Autodesk Inventor part; units mm, degrees
ref_plane "YZ Plane" through (0, 0, 0) normal (1, 0, 0) x (0, 1, 0)
ref_plane "XZ Plane" through (0, 0, 0) normal (0, 1, 0) x (-1, 0, 0)
ref_plane "XY Plane" through (0, 0, 0) normal (0, 0, 1) x (1, 0, 0)
sketch "main" plane through (0, 0, 0) normal (0, 0, 1) x (1, 0, 0)
  line L0 (-49.2738, 43.4655) -> (65.0262, 43.4655)
  circle A0 centre (65.0262, 37.1155) radius 2.1844
  line L1 (71.3762, 37.1155) -> (71.3762, 32.7721)
  arc A1 (71.3762, 37.1155) -> (65.0262, 43.4655) centre (65.0262, 37.1155) ccw
  line L2 (-71.4988, 29.5971) -> (-102.2861, 29.5971)
  line L3 (-105.3112, 25.4581) -> (-94.5785, -8.22)
  line L4 (-58.7988, 29.5971) -> (118.0384, 29.5971)
  line L5 (121.0635, 25.4581) -> (110.3309, -8.22)
  line L6 (101.2556, -14.8529) -> (-85.5032, -14.8529)
  arc A2 (-94.5785, -8.22) -> (-85.5032, -14.8529) centre (-85.5032, -5.3279) ccw
  arc A3 (101.2556, -14.8529) -> (110.3309, -8.22) centre (101.2556, -5.3279) ccw
  arc A4 (-102.2861, 29.5971) -> (-105.3112, 25.4581) centre (-102.2861, 26.4221) ccw
  arc A5 (121.0635, 25.4581) -> (118.0384, 29.5971) centre (118.0384, 26.4221) ccw
  arc A6 (71.3762, 32.7721) -> (74.5512, 29.5971) centre (74.5512, 32.7721) ccw
  line L7 (-58.7988, 29.5971) -> (-71.4988, 29.5971)
  circle A7 centre (-49.2738, 37.1155) radius 2.1844
  arc A8 (-49.2738, 43.4655) -> (-55.6238, 37.1155) centre (-49.2738, 37.1155) ccw
  line L8 (-55.6238, 37.1155) -> (-55.6238, 32.7721)
  arc A9 (-58.7988, 29.5971) -> (-55.6238, 32.7721) centre (-58.7988, 32.7721) ccw
  point P0 (1.5262, 9.2461)
  point P1 (-55.8302, 29.5971)
  point P2 (-106.6302, 29.5971)
  point P3 (-92.4647, -14.8529)
  point P4 (122.3826, 29.5971)
  point P5 (108.2171, -14.8529)
  dimension "d0" = 12.7
  dimension "d11" = 50.8
  dimension "d17" = 9.525
  dimension "d18" = 9.525
  dimension "d19" = 3.175
  dimension "d20" = 3.175
  dimension "d23" = 44.45
  dimension "d24" = 4.3688
  dimension "d25" = 186.7588
  dimension "d26" = 3.175
sketch "Sketch1" plane through (0, 0, 0) normal (0, 1, 0) x (-1, 0, 0)
  line L0 (-114.3, 6.35) -> (0, 6.35)
  circle A0 centre (0, 0) radius 2.1844
  line L1 (6.35, 0) -> (6.35, -4.3434)
  arc A1 (6.35, 0) -> (0, 6.35) centre (0, 0) ccw
  line L2 (-136.525, -7.5184) -> (-167.3123, -7.5184)
  line L3 (-170.3374, -11.6575) -> (-159.6047, -45.3356)
  line L4 (-123.825, -7.5184) -> (53.0123, -7.5184)
  line L5 (56.0374, -11.6575) -> (45.3047, -45.3356)
  line L6 (36.2294, -51.9684) -> (-150.5294, -51.9684)
  arc A2 (-159.6047, -45.3356) -> (-150.5294, -51.9684) centre (-150.5294, -42.4434) ccw
  arc A3 (36.2294, -51.9684) -> (45.3047, -45.3356) centre (36.2294, -42.4434) ccw
  arc A4 (-167.3123, -7.5184) -> (-170.3374, -11.6575) centre (-167.3123, -10.6934) ccw
  arc A5 (56.0374, -11.6575) -> (53.0123, -7.5184) centre (53.0123, -10.6934) ccw
  arc A6 (6.35, -4.3434) -> (9.525, -7.5184) centre (9.525, -4.3434) ccw
  line L7 (-123.825, -7.5184) -> (-136.525, -7.5184)
  circle A7 centre (-114.3, 0) radius 2.1844
  arc A8 (-114.3, 6.35) -> (-120.65, 0) centre (-114.3, 0) ccw
  line L8 (-120.65, 0) -> (-120.65, -4.3434)
  arc A9 (-123.825, -7.5184) -> (-120.65, -4.3434) centre (-123.825, -4.3434) ccw
extrude "Extrusion1" add sketch "Sketch1" along normal blind 1.5875
feature "Bend Part2" [suppressed]
equation "\"BendRadius\" = Thickness"
equation "\"BendReliefWidth\" = Thickness"
equation "\"BendReliefDepth\" = 0.5 * Thickness"
equation "\"CornerReliefSize\" = 4 * Thickness"
equation "\"MinimumRemnant\" = 2 * Thickness"
equation "\"TransitionRadius\" = BendRadius"
equation "\"JacobiRadiusSize\" = BendRadius"
equation "\"GapSize\" = Thickness"
properties part number "intake_wedge" material "Acetal Resin, White"
Model file for the job. Use its own axes, mm. Coordinates: 2 decimals unless noted, no trailing zeros. Order: outer loops, then holes, each group sorted by start corner. A loop starts at its lowest first (then second) coordinate and runs counter-clockwise, first axis right, second up. Notation, with made-up numbers: M -19.75,-39 L 26.25,-39 A32 ccw 26.25,-8 Z; hole C 48.25,-12 d7. An arc over 180 degrees is marked long. Return JSON: item names as keys, results as strings.
1. Saw through at C-C (x = 153). Give the cut face in (y, z).
Ans:
{"outline": "M 0,-51.64 L 1.59,-51.64 L 1.59,-7.52 L 0,-7.52 Z"}
2. Saw through at B-B (z = -19). Give the cut face in (x, y).
Ans:
{"outline": "M -53.7,0 L 168,0 L 168,1.59 L -53.7,1.59 Z"}
3. Flat gauge pins, fed straight in: pin 1 (0.8 mm diameter, centred on y = 1, z = -1.5, fed in from -X); pin 2 (5.5 mm diameter, centred on x = 0, z = 0, fed in from -Y); pin 3 (0.5 mm diameter, centred on y = 0.5, z = -3, fed in from +X). Where does each tip first touch, or does it go through?
Ans:
{"pin 1": "x = -6.35", "pin 2": "y = 0", "pin 3": "x = 120.65"}
4. Saw through at A-A (y = 0.4). Give the number of separate pieces and of enclosed holes in the cut face, and give its area (3 significant figures).
Ans:
{"separate pieces": "1", "enclosed holes": "2", "area": "11,200 mm^2"}
5. Pull direction Z, two halves, no side cores. Call faces 1 (the face through (118.84, 0.78, 4.44)), 2 (the face through (-2.084, 0.783, -0.656)), 3 (the face through (-41.92, 0.78, -50.08)), 4 (the face through (59, 0, -22)): +Z half, -Z half, draft (parallel to the pull), parting line (faces both ways), or undercut.
Ans:
{"face 1": "+Z half", "face 2": "undercut", "face 3": "-Z half", "face 4": "draft"}
6. Drill centre lines: probe 1 along Z at (x, y) = (0, 0.95); probe 2 along X at (y, z) = (0.65, -11.5). Where is each one in solid material? Low to high.
Ans:
{"probe 1": "-51.97 to -2.18, 2.18 to 6.35", "probe 2": "-56.08 to 170.38"}
